from build123d import *

# Parameters (mm, degrees)
SKETCH1_W           = 12.7
SKETCH1_H           = 19.05
SKETCH1_R           = 3.81
BOSS_EXTRUDE1_DEPTH = 1.778
FILLET1_R           = 0.508


with BuildPart() as part:
    # Sketch1 → Boss-Extrude1 (new body)
    with BuildSketch(Plane(origin=(0, 0, 0), x_dir=(0, 0, -1), z_dir=(1, 0, 0))):
        Rectangle(SKETCH1_W, SKETCH1_H)
        Circle(SKETCH1_R, mode=Mode.SUBTRACT)
    extrude(amount=BOSS_EXTRUDE1_DEPTH)

    # Fillet1
    fillet1_edges = [part.edges().sort_by_distance(p)[0] for p in [
        (0, 0, 3.81),
        (1.778, 0, 3.81),
        (1.778, 0, 6.35),
        (1.778, -9.525, 0),
        (1.778, 0, -6.35),
        (0, -9.525, 0),
        (0, 0, 6.35),
        (0, 9.525, 0),
        (0, 0, -6.35),
        (1.778, 9.525, 0),
    ]]
    fillet(fillet1_edges, radius=FILLET1_R)


solid = part.part
Read the model definition and answer for the solid it produces. Units are mm, in the model's axes. Coordinates: 2 decimals unless noted, no trailing zeros. Loops run counter-clockwise (first coordinate to the right, second up) from the corner with the lowest first, then second, coordinate; pieces in that order, holes last. Notation, with made-up numbers: (-35, 9.25) - (-18, 9.25) arc R11 ccw to (-18, 22.25) - close; hole circle Ø4 at (-23.75, 8). An arc over 180 degrees is marked (long way). Answer in a Markdown table with one row per item.
Q1. Find section B-B on y = 0. Write down the section's boundary in (x, z), plus the area to 3 significant figures.
Here are the results:
| item | result |
|---|---|
| outline | (0, -5.84) arc R0.51 ccw to (0.51, -6.35) - (1.27, -6.35) arc R0.51 ccw to (1.78, -5.84) - (1.78, -4.32) arc R0.51 ccw to (1.27, -3.81) - (0.51, -3.81) arc R0.51 ccw to (0, -4.32) - close; (0, 4.32) arc R0.51 ccw to (0.51, 3.81) - (1.27, 3.81) arc R0.51 ccw to (1.78, 4.32) - (1.78, 5.84) arc R0.51 ccw to (1.27, 6.35) - (0.51, 6.35) arc R0.51 ccw to (0, 5.84) - close |
| area | 8.59 mm^2 |
Q2. Find section A-A on z = 0. Write down the section's boundary in (x, y) (3 decimals).
Here are the results:
| item | result |
|---|---|
| outline | (0, -9.017) arc R0.508 ccw to (0.508, -9.525) - (1.27, -9.525) arc R0.508 ccw to (1.778, -9.017) - (1.778, -4.318) arc R0.508 ccw to (1.27, -3.81) - (0.508, -3.81) arc R0.508 ccw to (0, -4.318) - close; (0, 4.318) arc R0.508 ccw to (0.508, 3.81) - (1.27, 3.81) arc R0.508 ccw to (1.778, 4.318) - (1.778, 9.017) arc R0.508 ccw to (1.27, 9.525) - (0.508, 9.525) arc R0.508 ccw to (0, 9.017) - close |
Q3. The mould has two halves that part along Z. Classify faces 1 (the cylindrical face through (0.88, -3.72, 0.83)), 2 (the flat face through (1.778, 2, 4)): pulls with the +Z half, pulls with the -Z half, needs draft (parallel to the pull), parting line crosses it, or undercut.
Here are the results:
| item | result |
|---|---|
| face 1 | undercut |
| face 2 | needs draft |
Q4. Straight lines are drawn through the part: line 1 along Y through (x, z) = (0.8, 0) (3 decimals); line 2 along Z through (x, y) = (0.8, 0.75); line 3 along Y through (x, z) = (1.3, -2.5). For each, find the intervals that lie inside material, in ascending order. Write a range as [from, to].
Here are the results:
| item | result |
|---|---|
| line 1 | y = [-9.525, -3.81], [3.81, 9.525] |
| line 2 | z = [-6.35, -3.74], [3.74, 6.35] |
| line 3 | y = [-9.52, -2.88], [2.88, 9.52] |
